Autodesk Inventor part; units mm, degrees
ref_plane "YZ Plane" through (0, 0, 0) normal (1, 0, 0) x (0, 1, 0)
ref_plane "XZ Plane" through (0, 0, 0) normal (0, 1, 0) x (-1, 0, 0)
ref_plane "XY Plane" through (0, 0, 0) normal (0, 0, 1) x (1, 0, 0)
sketch "Sketch1" plane through (0, 0, 0) normal (0, 0, 1) x (1, 0, 0)
  line L0 (-10, -5) -> (10, -5)
  line L1 (10, -5) -> (10, 5)
  line L2 (10, 5) -> (-10, 5)
  line L3 (-10, 5) -> (-10, -5)
  line L4 (-10, -5) -> (10, 5) construction
  line L5 (10, -5) -> (-10, 5) construction
  line L6 (-14, 0) -> (14, 0) construction
  circle A0 centre (3.75, 0) radius 1.5
  point P0 (0, 0)
  dimension "d0" = 20
  dimension "d1" = 10
  dimension "d2" = 3
  dimension "d3" = 3.75
extrude "Extrusion1" add sketch "Sketch1" along normal blind 6.65
sketch "Sketch2" plane through (0, 0, 6.65) normal (0, 0, 1) x (1, 0, 0)
  line L0 (-14, 0) -> (14, 0)
  circle A0 centre (-3.75, 0) radius 1.4
  point P0 (0, 0)
  dimension "d6" = 2.8
  dimension "d7" = 3.75
extrude "Extrusion2" add sketch "Sketch2" along normal blind 2
fillet "Fillet2" radius 1 4 edges at (10, -5, 3.325) (10, 5, 3.325) (-10, -5, 3.325) (-10, 5, 3.325)
properties part number "PWR_PCBA_HeatSink"
Geometry: final body of the model. Coordinates: model frame, mm. A direction names the side the tool comes from. Round coordinates to 2 decimals unless told otherwise and drop trailing zeros. Order: outer loops, then holes, each group sorted by start corner. A loop starts at its lowest first (then second) coordinate and runs counter-clockwise, first axis right, second up. Notation, with made-up numbers: M 68,74.5 L 88,74.5 A25 cw 88,105.5 Z; hole C 47.5,42 d1. An arc over 180 degrees is marked long. One line per item, written item: value.
(1) Reachability of faces 1 (the cylindrical face through (9.715, 4.699, 3.372)), 2 (the cylindrical face through (-2.415, -0.421, 7.636)) from +Z, -Z, +X, -X, +Y, -Y: full face, straight path, thin tool, end or side. Return the list, or none.
Result sheet:
face 1: +Z, -Z, +X, +Y
face 2: +Z
(2) Cut plane B-B (z = 1). Return the cut outline in (x, y).
Result sheet:
outline: M -10,-4 A1 ccw -9,-5 L 9,-5 A1 ccw 10,-4 L 10,4 A1 ccw 9,5 L -9,5 A1 ccw -10,4 Z; hole C 3.75,0 d3
(3) Cut plane D-D (x = -3.75). Return the cut outline in (y, z), and give its area (3 significant figures).
Result sheet:
outline: M -5,0 L 5,0 L 5,6.65 L 1.4,6.65 L 1.4,8.65 L -1.4,8.65 L -1.4,6.65 L -5,6.65 Z
area: 72.1 mm2
(4) Cut plane C-C (x = 3.75). Return the cut outline in (y, z).
Result sheet:
outline: M -5,0 L -1.5,0 L -1.5,6.65 L -5,6.65 Z; M 1.5,0 L 5,0 L 5,6.65 L 1.5,6.65 Z
(5) Cut plane A-A (y = 0). Return the cut outline in (x, z), and give its area (3 significant figures).
Result sheet:
outline: M -10,0 L 2.25,0 L 2.25,6.65 L -2.35,6.65 L -2.35,8.65 L -5.15,8.65 L -5.15,6.65 L -10,6.65 Z; M 5.25,0 L 10,0 L 10,6.65 L 5.25,6.65 Z
area: 119 mm2
(6) Pull-direction query (Y, two-part tool) for faces 3 (the cylindrical face through (5.136, 0.575, 3.278)), 4 (the flat face through (0, 5, 3)), 5 (the cylindrical face through (-9.715, -4.699, 3.372)), 6 (the flat face through (-4, 0, 8.65)); classes: pulls with the +Y half, pulls with the -Y half, needs draft (parallel to the pull), parting line crosses it, or undercut.
Result sheet:
face 3: undercut
face 4: pulls with the +Y half
face 5: pulls with the -Y half
face 6: needs draft
(7) Pin query (flat end, axial travel): P1, Ø4, axis at x = 3.75, y = 0, coming from the +Z side. Return the tip coordinate at first contact, or that it passes through.
Result sheet:
P1: z = 6.65
(8) Line query: probe 1 along Y at (x, z) = (3.75, 2.25); probe 2 along Z at (x, y) = (-6.25, 0.25). Output: solid intervals per line, ascending. Write a range as [from, to].
Result sheet:
probe 1: [-5, -1.5], [1.5, 5]
probe 2: [0, 6.65]
